Could you check a few things on this model? Use its own coordinates, in mm. Face numbers are marked on the shaded views. Give positions to 0.01 mm unless a question says otherwise; leave off trailing zeros. Loops run counter-clockwise (first coordinate to the right, second up) from the corner with the lowest first, then second, coordinate; pieces in that order, holes last. Notation, with made-up numbers: M 32,1.25 L 83,1.25 A23 ccw 83,17.25 Z; hole C 20,-11.75 d8. An arc over 180 degrees is marked long. Answer in a Markdown table with one row per item. Add a question column.
```python
from build123d import *

# Parameters (mm, degrees)
HOOK_DEPTH          = 3
SKETCH2_W           = 70
SKETCH2_H           = 3.5
PIN_DEPTH           = 3
CUT_EXTRUDE1_DEPTH  = 3.5
FILLET1_R           = 0.5
SKETCH4_W           = 10
SKETCH4_H           = 10
BOSS_EXTRUDE3_DEPTH = 0.2


with BuildPart() as part:
    # Sketch1 → Hook (new body)
    with BuildSketch(Plane.XY):
        with BuildLine():
            Line((1, -11), (-3, -11))
            Line((-3, -11), (-7.5, -11))
            Line((-7.5, -11), (-7.5, -10))
            Line((-7.5, -10), (-3, -10))
            Line((-3, -10), (-3, 10))
            Line((-3, 10), (-7.5, 10))
            Line((-7.5, 10), (-7.5, 11))
            Line((-7.5, 11), (-3, 11))
            Line((-3, 11), (1, 11))
            ThreePointArc((1, 11), (2.414213562, 10.414213562), (3, 9))
            Line((3, 9), (3, 8.408634703))
            ThreePointArc((3, 8.408634703), (2.961405113, 8.017623214), (2.847110016, 7.64170277))
            ThreePointArc((2.847110016, 7.64170277), (1.32371561, 0), (2.847110016, -7.64170277))
            ThreePointArc((2.847110016, -7.64170277), (2.961405113, -8.017623214), (3, -8.408634703))
            Line((3, -8.408634703), (3, -9))
            ThreePointArc((3, -9), (2.414213562, -10.414213562), (1, -11))
        make_face()
        with BuildLine():
            Line((2, 8.9), (2, 9.1))
            ThreePointArc((2, 9.1), (1.736396103, 9.736396103), (1.1, 10))
            Line((1.1, 10), (0, 10))
            ThreePointArc((0, 10), (-1.414213562, 9.414213562), (-2, 8))
            Line((-2, 8), (-2, -8))
            ThreePointArc((-2, -8), (-1.414213562, -9.414213562), (0, -10))
            Line((0, -10), (1.1, -10))
            ThreePointArc((1.1, -10), (1.736396103, -9.736396103), (2, -9.1))
            Line((2, -9.1), (2, -8.9))
            ThreePointArc((2, -8.9), (1.736396103, -8.263603897), (1.1, -8))
            Line((1.1, -8), (0.9, -8))
            ThreePointArc((0.9, -8), (0.263603897, -7.736396103), (0, -7.1))
            Line((0, -7.1), (0, 7.1))
            ThreePointArc((0, 7.1), (0.263603897, 7.736396103), (0.9, 8))
            Line((0.9, 8), (1.1, 8))
            ThreePointArc((1.1, 8), (1.736396103, 8.263603897), (2, 8.9))
        make_face(mode=Mode.SUBTRACT)
    extrude(amount=HOOK_DEPTH)

    # Sketch2 → Pin (add)
    with BuildSketch(Plane.XY):
        with Locations((35, 5)):
            Rectangle(SKETCH2_W, SKETCH2_H)
    extrude(amount=PIN_DEPTH)

    # Sketch3 → Cut-Extrude1 (cut)
    with BuildSketch(Plane.XZ.offset(-3.25)):
        Polygon((62, 3), (70, 3), (70, 1), align=None)
    extrude(amount=-CUT_EXTRUDE1_DEPTH, mode=Mode.SUBTRACT)

    # Fillet1
    fillet1_edges = [part.edges().sort_by_distance(p)[0] for p in [
        (70, 5, 0),
        (70, 5, 1),
    ]]
    fillet(fillet1_edges, radius=FILLET1_R)

    # Sketch4 → Boss-Extrude3 (add)
    with BuildSketch(Plane.XY):
        with Locations((54.047822984, -1.75)):
            Rectangle(SKETCH4_W, SKETCH4_H)
    extrude(amount=BOSS_EXTRUDE3_DEPTH)


solid = part.part
```
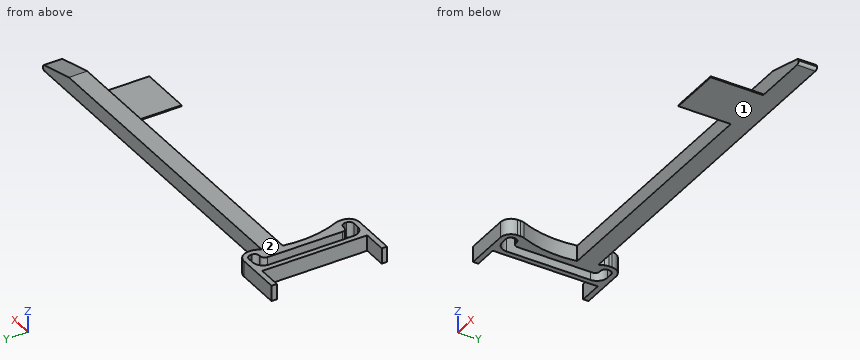
Item 1: Suppose I cut it at D-D (x = 63). List the corners of the cut face in (y, z) for me.
Item 2: For P1, Ø5, axis at x = 53.5, y = -3.5, coming from the +Z side; P2, Ø0.9, axis at x = 43.5, z = 1, coming from the +Y side, each with a flat end and sliding along its axis, tell me the tip position at first contact or that it passes through.
Item 3: I need wall thicknesses on L1, parallel to Y at x = 1, z = 2.1; L2, parallel to X at y = -0.5, z = 1.7; L3, parallel to Y at x = 21, z = 1.35. Which ranges of each line are inside material? Lowest first, please.
Item 4: Suppose I cut it at A-A (y = 5.75). List the corners of the cut face in (x, z) for me, then the cut area to 3 significant figures.
Item 5: If we mould it in two halves opening along Z, with no side actions, what happens to the marked faces 1 and 2? For each: +Z half, -Z half, draft (parallel to the pull), parting line (faces both ways), or undercut.
Item 6: Suppose I cut it at C-C (y = -1.5). List the corners of the cut face in (x, z) for me.
Values found:
| question | item | result |
|---|---|---|
| 1 | outline | M 3.25,0 L 6.75,0 L 6.75,2.75 L 3.25,2.75 Z |
| 2 | P1 | z = 0.2 |
| 2 | P2 | y = 6.75 |
| 3 | L1 | -11 to -10, -8 to 8, 10 to 11 |
| 3 | L2 | -3 to -2, 0 to 1.33 |
| 3 | L3 | 3.25 to 6.75 |
| 4 | outline | M -3,0 L -2,0 L -2,3 L -3,3 Z; M 0,0 L 69.5,0 A0.5 ccw 70,0.5 L 70,0.61 A0.5 ccw 69.62,1.09 L 62,3 L 0,3 Z |
| 4 | area | 205 mm² |
| 5 | face 1 | -Z half |
| 5 | face 2 | +Z half |
| 6 | outline | M -3,0 L -2,0 L -2,3 L -3,3 Z; M 0,0 L 1.38,0 L 1.38,3 L 0,3 Z; M 49.05,0 L 59.05,0 L 59.05,0.2 L 49.05,0.2 Z |
